Job drawing, mm, ordinate dimensions from the low corner. One solid piece. A direction names the side the tool comes from. Round coordinates to 2 decimals unless told otherwise and drop trailing zeros. Loops run counter-clockwise (first coordinate to the right, second up) from the corner with the lowest first, then second, coordinate; pieces in that order, holes last.
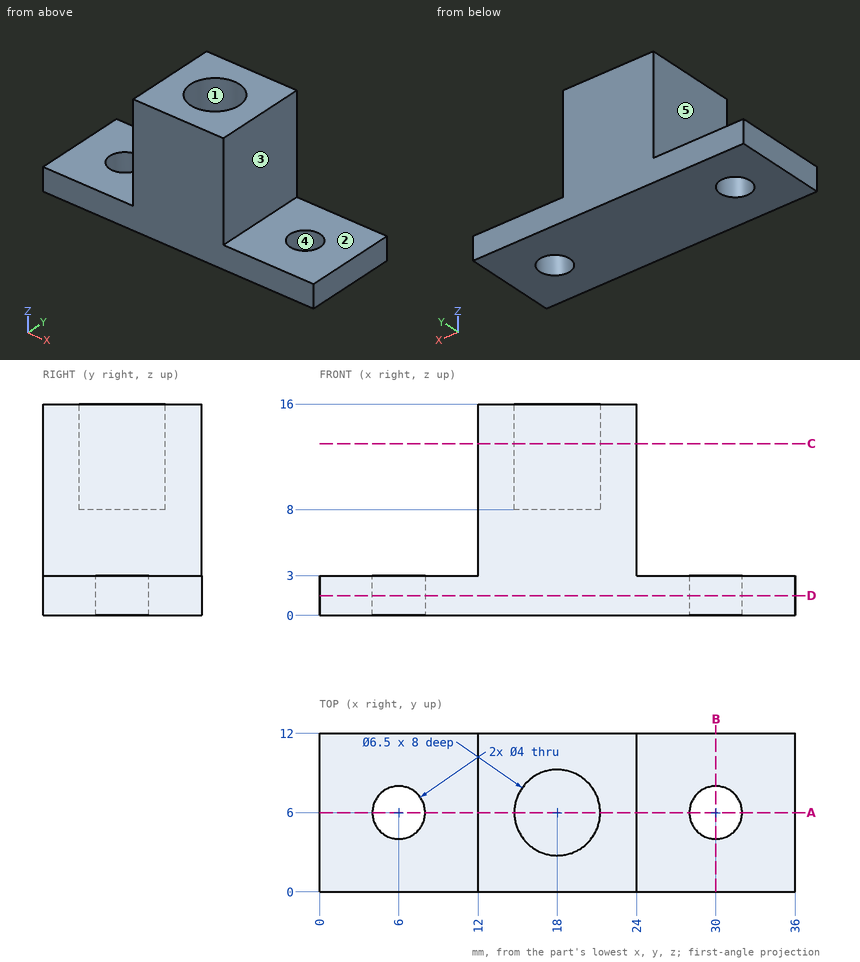
(1) Slice it at A-A on y = 6. List the corners of the cut face in (x, z).
Responses:
outline: (0, 0) - (4, 0) - (4, 3) - (0, 3) - close; (8, 0) - (28, 0) - (28, 3) - (24, 3) - (24, 16) - (21.25, 16) - (21.25, 8) - (14.75, 8) - (14.75, 16) - (12, 16) - (12, 3) - (8, 3) - close; (32, 0) - (36, 0) - (36, 3) - (32, 3) - close
(2) Probe line 1 (Y direction, x = 18, z = 11); line 2 (Z direction, x = 9, y = 5); line 3 (X direction, y = 3.25, z = 6). List the from-to ranges inside material, lowest first.
Responses:
line 1: y = 0 to 2.75, 9.25 to 12
line 2: z = 0 to 3
line 3: x = 12 to 24
(3) Slice it at D-D on z = 1.5. List the corners of the cut face in (x, y).
Responses:
outline: (0, 0) - (36, 0) - (36, 12) - (0, 12) - close; hole circle Ø4 at (6, 6); hole circle Ø4 at (30, 6)
(4) Pull direction X, two halves, no side cores. Call the marked faces 1, 2 and 3: +X half, -X half, draft (parallel to the pull), parting line (faces both ways), or undercut.
Responses:
face 1: undercut
face 2: draft
face 3: +X half
(5) Which spindle directions (+Z, -Z, +X, -X, +Y, -Y) get a long thin tool onto all of the face, cutting with end or side? Do the marked faces 4 and 5. Say none if no direction does.
Responses:
face 4: +Z, -Z
face 5: +Z, -X, +Y, -Y
(6) Pin check, flat tips, straight feed: P1, Ø6, axis at y = 9, z = 11.5, coming from the -X side; P2, Ø2, axis at x = 18.5, y = 7.5, coming from the +Z side; P3, Ø5, axis at x = 6, y = 6, coming from the +Z side. Stop position of each tip, or through.
Responses:
P1: stops at x = 12
P2: stops at z = 8
P3: stops at z = 3
(7) Slice it at B-B on x = 30. List the corners of the cut face in (y, z).
Responses:
outline: (0, 0) - (4, 0) - (4, 3) - (0, 3) - close; (8, 0) - (12, 0) - (12, 3) - (8, 3) - close
(8) Slice it at C-C on z = 13. List the corners of the cut face in (x, y).
Responses:
outline: (12, 0) - (24, 0) - (24, 12) - (12, 12) - close; hole circle Ø6.5 at (18, 6)
